Part model, mm, in its own coordinate system. A direction names the side the tool comes from. Give positions to 0.01 mm unless a question says otherwise; leave off trailing zeros. Write each loop counter-clockwise with the first axis right and the second up, starting at its lowest first coordinate (ties: lowest second). Pieces come first, ordered by that corner, then holes. Notation, with made-up numbers: M 78.25,0 L 101.25,0 A25 cw 101.25,30 Z; hole C 14,47 d6. An arc over 180 degrees is marked long. Answer as CSV lines item,"result". Start each with the question number.
1) Mould opens along X. For faces 4 (the flat face through (0, -1.27, 3)), 5 (the flat face through (-4.964, 0, -8)), 6 (the cylindrical face through (-0.49, -0.02, -15.81)) say: pulls with the +X half, pulls with the -X half, needs draft (parallel to the pull), parting line crosses it, or undercut.
2) Pin check, flat tips, straight feed: pin 1 Ø1.5 at (x, y) = (7, 0.5) entering from -Z; pin 2 Ø0.8 at (y, z) = (0.5, -4.5) entering from -X; pin 3 Ø0.8 at (y, z) = (0.5, -9) entering from +X. Stop position of each tip, or through.
3) Slice it at B-B, the plane y = 0.45. Give the cut face in (x, z).
4) Slice it at D-D, the plane x = 8.5. Give the cut face in (y, z), plus the area to 3 significant figures.
5) Wall check: line 1 along X through (y, z) = (0.85, -17); line 2 along X through (y, z) = (-0.7, -12.5); line 3 along Z through (x, y) = (11.5, 0.65). Give the ranges that are in metal, low to high. Write a range as from..to.
6) Slice it at C-C, the plane z = -4. Give the cut face in (x, y).
7) Slice it at A-A, the plane x = 0. Give the cut face in (y, z).
8) Tool access for faces 1 (the flat face through (-15, 0, 0)), 2 (the flat face through (-25.565, 0, 6)), 3 (the flat face through (4.964, 0, -9)): list every direction of +Z, -Z, +X, -X, +Y, -Y with a clear straight run to the whole face (end or side of a thin tool).
```python
from build123d import *

# Parameters (mm, degrees)
SKETCH1_R           = 1.27
BOSS_EXTRUDE1_DEPTH = 1.27


with BuildPart() as part:
    # Sketch1 → Boss-Extrude1 (new, symmetric)
    with BuildSketch(Plane(origin=(0, 0, 0), x_dir=(1, 0, 0), z_dir=(0, 1, 0))):
        with BuildLine():
            Line((4.963813713, 0), (25.565066873, 0))
            Line((25.565066873, 0), (25.565066873, -12.782533436))
            Line((25.565066873, -12.782533436), (-25.565066873, -12.782533436))
            Line((-25.565066873, -12.782533436), (-25.565066873, 0))
            Line((-25.565066873, 0), (-4.963813713, 0))
            Line((-4.963813713, 0), (-4.963813713, 16.980141079))
            ThreePointArc((-4.963813713, 16.980141079), (0, 21.943954793), (4.963813713, 16.980141079))
            Line((4.963813713, 16.980141079), (4.963813713, 0))
        make_face()
        with Locations(Location((0, 16.980141079, 0), (0, 0, 270))):
            Circle(SKETCH1_R, mode=Mode.SUBTRACT)
    extrude(amount=BOSS_EXTRUDE1_DEPTH, both=True)


solid = part.part
```
Found:
1,face 4,"needs draft"
1,face 5,"pulls with the -X half"
1,face 6,"undercut"
2,pin 1,"z = 0"
2,pin 2,"x = -4.96"
2,pin 3,"x = 4.96"
3,outline,"M -25.57,0 L -4.96,0 L -4.96,-16.98 A4.96 ccw 4.96,-16.98 L 4.96,0 L 25.57,0 L 25.57,12.78 L -25.57,12.78 Z; hole C 0,-16.98 d2.54"
4,outline,"M -1.27,0 L 1.27,0 L 1.27,12.78 L -1.27,12.78 Z"
4,area,"32.5 mm²"
5,line 1,"-4.96..-1.27, 1.27..4.96"
5,line 2,"-4.96..4.96"
5,line 3,"0..12.78"
6,outline,"M -4.96,-1.27 L 4.96,-1.27 L 4.96,1.27 L -4.96,1.27 Z"
7,outline,"M -1.27,-21.94 L 1.27,-21.94 L 1.27,-18.25 L -1.27,-18.25 Z; M -1.27,-15.71 L 1.27,-15.71 L 1.27,12.78 L -1.27,12.78 Z"
8,face 1,"-Z, -X, +Y, -Y"
8,face 2,"+Z, -Z, -X, +Y, -Y"
8,face 3,"-Z, +X, +Y, -Y"
